```python
from build123d import *

# Parameters (mm, degrees)
SKETCH2_W           = 21
SKETCH2_H           = 36
BOSS_EXTRUDE1_DEPTH = 10
BOSS_EXTRUDE2_DEPTH = 30


with BuildPart() as part:
    # Sketch2 → Boss-Extrude1 (new body)
    with BuildSketch(Plane(origin=(0, 0, 0), x_dir=(1, 0, 0), z_dir=(0, 1, 0))):
        with BuildLine():
            Line((67.865, 0), (45, 0))
            Line((45, 0), (45, -22.5))
            Line((45, -22.5), (14, -22.5))
            Line((14, -22.5), (14, 12.5))
            Line((14, 12.5), (-14, 12.5))
            Line((-14, 12.5), (-14, -22.5))
            Line((-14, -22.5), (-40, -22.5))
            Line((-40, -22.5), (-40, -17.5))
            Line((-40, -17.5), (-19, -17.5))
            Line((-19, -17.5), (-19, 18.5))
            Line((-19, 18.5), (0, 18.5))
            Line((0, 18.5), (0, 61.5))
            Line((0, 61.5), (-28.695090608, 61.5))
            ThreePointArc((-28.695090608, 61.5), (36.457275686, 57.240940546), (67.865, 0))
        make_face()
        with Locations((29.5, 0.5)):
            Rectangle(SKETCH2_W, SKETCH2_H, mode=Mode.SUBTRACT)
    extrude(amount=BOSS_EXTRUDE1_DEPTH)

    # Sketch3 → Boss-Extrude2 (add)
    with BuildSketch(Plane.XZ):
        Polygon((0, -61.5), (0, -67.865), (-2.244041558, -67.827888825), (-17.609918894, -65.540437758), (-28.695090608, -61.5), align=None)
    extrude(amount=BOSS_EXTRUDE2_DEPTH)


solid = part.part
```
The model under review builds one solid part; all positions refer to its coordinate system, in mm. A direction names the side the tool comes from. Round coordinates to 2 decimals unless told otherwise and drop trailing zeros. Order: outer loops, then holes, each group sorted by start corner. A loop starts at its lowest first (then second) coordinate and runs counter-clockwise, first axis right, second up. Notation, with made-up numbers: (81.5, 24.5) -> (88.5, 24.5) arc R20 ccw to (88.5, 63.5) -> close; hole circle Ø6 at (44.25, -23). An arc over 180 degrees is marked (long way). One line per item, written item: value. Start each with the question number.
Q1. Take a section at D-D (y = -19). Write out the cut boundary in (x, z) (3 decimals), and give its area (3 significant figures).
Q2. Mouldability with a two-part tool opening along Z and no side actions: class faces 1 (the face through (57, 5, 0)), 2 (the face through (-14, 5, 5)), 3 (the face through (0, 5, -40)), 4 (the face through (29, 5, -18.5)) as released by +Z, released by -Z, zero draft, split by the parting line, or undercut.
Q3. Take a section at B-B (y = 6.5). Write out the cut boundary in (x, z) (3 decimals), and give its area (3 significant figures).
Q4. Take a section at A-A (z = 3.5). Write out the cut boundary in (x, y), and give its area (3 significant figures).
Q5. Clearance check with flat-ended pins moving along their axes: pin 1 Ø8 at (y, z) = (5.5, 7) entering from -X; pin 2 Ø11 at (x, y) = (-34.5, 6.5) entering from -Z; pin 3 Ø3 at (y, z) = (6, -8.5) entering from +X; pin 4 Ø12 at (x, y) = (-28.5, -1.5) entering from +Z. State where each tip first meets the part, or that it passes through.
Q6. Wall thickness on line 1 (Y direction, x = 54.5, z = -2); line 2 (X direction, y = 3, z = -11); line 3 (Z direction, x = -7, y = -14): over which ranges is each line inside the solid? List them lowest first.
Q7. Machinability: for faces 5 (the face through (0, -15, -65)), 6 (the face through (-30, 5, 17.5)), 7 (the face through (29, 5, 17.5)), which of the approach directions +Z, -Z, +X, -X, +Y, -Y give a long, thin tool a straight path to every point of the face, cutting with its end or side? Answer none if there is none.
Q8. Take a section at C-C (x = -5.5). Write out the cut boundary in (y, z), and give its area (3 significant figures).
Reported:
1. outline: (-28.695, -61.5) -> (-17.61, -65.54) -> (-2.244, -67.828) -> (0, -67.865) -> (0, -61.5) -> close
1. area: 116 mm2
2. face 1: released by +Z
2. face 2: zero draft
2. face 3: undercut
2. face 4: undercut
3. outline: (-40, 17.5) -> (-19, 17.5) -> (-19, -18.5) -> (0, -18.5) -> (0, -61.5) -> (-28.695, -61.5) arc R67.865 ccw to (67.865, 0) -> (45, 0) -> (45, 22.5) -> (14, 22.5) -> (14, -12.5) -> (-14, -12.5) -> (-14, 22.5) -> (-40, 22.5) -> close; hole (19, -18.5) -> (40, -18.5) -> (40, 17.5) -> (19, 17.5) -> close
3. area: 3,900 mm2
4. outline: (-19, 0) -> (-14, 0) -> (-14, 10) -> (-19, 10) -> close; (14, 0) -> (19, 0) -> (19, 10) -> (14, 10) -> close; (40, 0) -> (45, 0) -> (45, 10) -> (40, 10) -> close
4. area: 150 mm2
5. pin 1: stops at x = -19
5. pin 2: stops at z = 17.5
5. pin 3: stops at x = 67.5
5. pin 4: stops at z = 22.5
6. line 1: y = 0 to 10
6. line 2: x = -19 to -14, 14 to 19, 40 to 66.97
6. line 3: z = -67.12 to -61.5
7. face 5: +Z, -Z, +X, -Y
7. face 6: -X, +Y, -Y
7. face 7: +Y, -Y
8. outline: (-30, -67.34) -> (0, -67.34) -> (0, -67.64) -> (10, -67.64) -> (10, -61.5) -> (-30, -61.5) -> close; (0, -18.5) -> (10, -18.5) -> (10, -12.5) -> (0, -12.5) -> close
8. area: 297 mm2
